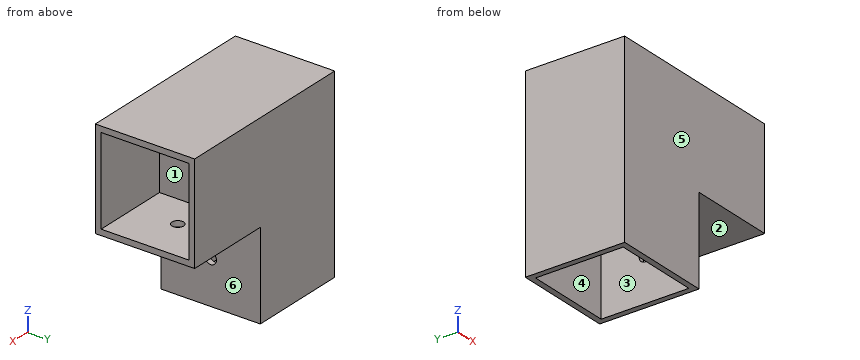
```python
from build123d import *

# Parameters (mm, degrees)
BOSS_EXTRUDE1_DEPTH = 51
SKETCH2_W           = 45
SKETCH2_H           = 45
CUT_EXTRUDE1_DEPTH  = 40
SKETCH3_W           = 45
SKETCH3_H           = 45
CUT_EXTRUDE2_DEPTH  = 40
CUT_EXTRUDE3_REACH  = 119.69
SKETCH4_R           = 3
CUT_EXTRUDE4_REACH  = 119.69
SKETCH5_R           = 3


with BuildPart() as part:
    # Sketch1 → Boss-Extrude1 (new body)
    with BuildSketch(Plane(origin=(0, 0, 0), x_dir=(1, 0, 0), z_dir=(0, 1, 0))):
        Polygon((-3, -3), (-3, 93), (48, 93), (48, 48), (93, 48), (93, -3), align=None)
    extrude(amount=BOSS_EXTRUDE1_DEPTH)

    # Sketch2 → Cut-Extrude1 (cut)
    with BuildSketch(Plane(origin=(93, 0, 0), x_dir=(0, 0, -1), z_dir=(1, 0, 0))):
        with Locations((22.5, 25.5)):
            Rectangle(SKETCH2_W, SKETCH2_H)
    extrude(amount=-CUT_EXTRUDE1_DEPTH, mode=Mode.SUBTRACT)

    # Sketch3 → Cut-Extrude2 (cut)
    with BuildSketch(Plane(origin=(0, 0, -93), x_dir=(-1, 0, 0), z_dir=(0, 0, -1))):
        with Locations((-22.5, 25.5)):
            Rectangle(SKETCH3_W, SKETCH3_H)
    extrude(amount=-CUT_EXTRUDE2_DEPTH, mode=Mode.SUBTRACT)

    # Sketch4 → Cut-Extrude3 (cut, up to next)
    with BuildSketch(Plane(origin=(0, 0, -48), x_dir=(-1, 0, 0), z_dir=(0, 0, -1)), mode=Mode.PRIVATE) as cut_extrude3_sk1:
        with Locations((-70.5, 25.5)):
            Circle(SKETCH4_R)
    cut_extrude3_tool1 = extrude(cut_extrude3_sk1.sketch, amount=-CUT_EXTRUDE3_REACH, mode=Mode.PRIVATE) & part.part
    add(cut_extrude3_tool1.solids().sort_by_distance((70.5, 25.5, -48))[0], mode=Mode.SUBTRACT)

    # Sketch5 → Cut-Extrude4 (cut, up to next)
    with BuildSketch(Plane(origin=(48, 0, 0), x_dir=(0, 0, -1), z_dir=(1, 0, 0)), mode=Mode.PRIVATE) as cut_extrude4_sk1:
        with Locations((70.5, 25.5)):
            Circle(SKETCH5_R)
    cut_extrude4_tool1 = extrude(cut_extrude4_sk1.sketch, amount=-CUT_EXTRUDE4_REACH, mode=Mode.PRIVATE) & part.part
    add(cut_extrude4_tool1.solids().sort_by_distance((48, 25.5, -70.5))[0], mode=Mode.SUBTRACT)


solid = part.part
```
Input: part model. Units: mm. Frame: model coordinates. Face numbers are marked on the shaded views. A direction names the side the tool comes from. Give positions to 0.01 mm unless a question says otherwise; leave off trailing zeros. Order: outer loops, then holes, each group sorted by start corner. A loop starts at its lowest first (then second) coordinate and runs counter-clockwise, first axis right, second up.
1. Line query: probe 1 along X at (y, z) = (46.5, -65); probe 2 along Y at (x, z) = (66, -10.5); probe 3 along Z at (x, y) = (64, 20). Output: solid intervals per line, ascending.
Computed:
probe 1: x = -3 to 0, 45 to 48
probe 2: y = 0 to 3, 48 to 51
probe 3: z = -48 to -45, 0 to 3
2. Set-up query: the marked faces 1, 2 and 3. Return all of +Z, -Z, +X, -X, +Y, -Y with unobstructed straight access to the full face (end or side cutting, diameter ignored); none if empty.
Computed:
face 1: +X
face 2: -Z, +X, +Y, -Y
face 3: -Z
3. Cut plane B-B (z = -76). Return loops of the section in (x, y).
Computed:
outline: (-3, 0) - (48, 0) - (48, 51) - (-3, 51) - close; hole (0, 3) - (45, 3) - (45, 48) - (0, 48) - close
4. Draft query along Y for the marked faces 4, 5 and 6. Return one class per face: released by +Y, released by -Y, zero draft, split by the parting line, or undercut.
Computed:
face 4: undercut
face 5: released by -Y
face 6: zero draft
5. Cut plane D-D (y = 11.5). Return loops of the section in (x, z).
Computed:
outline: (-3, -93) - (0, -93) - (0, -53) - (45, -53) - (45, -93) - (48, -93) - (48, -48) - (93, -48) - (93, -45) - (53, -45) - (53, 0) - (93, 0) - (93, 3) - (-3, 3) - close
6. Cut plane A-A (y = 25.5). Return loops of the section in (x, z), and give its area (4 significant figures).
Computed:
outline: (-3, -93) - (0, -93) - (0, -53) - (45, -53) - (45, -67.5) - (48, -67.5) - (48, -48) - (67.5, -48) - (67.5, -45) - (53, -45) - (53, 0) - (93, 0) - (93, 3) - (-3, 3) - close; (45, -93) - (48, -93) - (48, -73.5) - (45, -73.5) - close; (73.5, -48) - (93, -48) - (93, -45) - (73.5, -45) - close
area: 3,555 mm2
7. Cut plane C-C (x = 77.5). Return loops of the section in (y, z).
Computed:
outline: (0, -48) - (51, -48) - (51, 3) - (0, 3) - close; hole (3, -45) - (48, -45) - (48, 0) - (3, 0) - close
8. Pin query (flat end, axial travel): pin 1 Ø13.5 at (x, y) = (65, 17.5) entering from -Z; pin 2 Ø22.5 at (y, z) = (18, -80.5) entering from +X; pin 3 Ø5.5 at (y, z) = (25.5, -70.5) entering from +X. Return the tip coordinate at first contact, or that it passes through.
Computed:
pin 1: stops at z = -48
pin 2: stops at x = 48
pin 3: stops at x = 0
